Verification items for this drawing (mm, ordinates from the low corner). Give positions to 0.01 mm unless a question says otherwise; leave off trailing zeros. Write each loop counter-clockwise with the first axis right and the second up, starting at its lowest first coordinate (ties: lowest second). Pieces come first, ordered by that corner, then holes. Notation, with made-up numbers: (27.5, 45.25) -> (78.5, 45.25) arc R22 cw to (78.5, 58.25) -> close; hole circle Ø6 at (64.5, -6). An arc over 180 degrees is marked (long way). Answer as a JSON object with one key per item and string values.
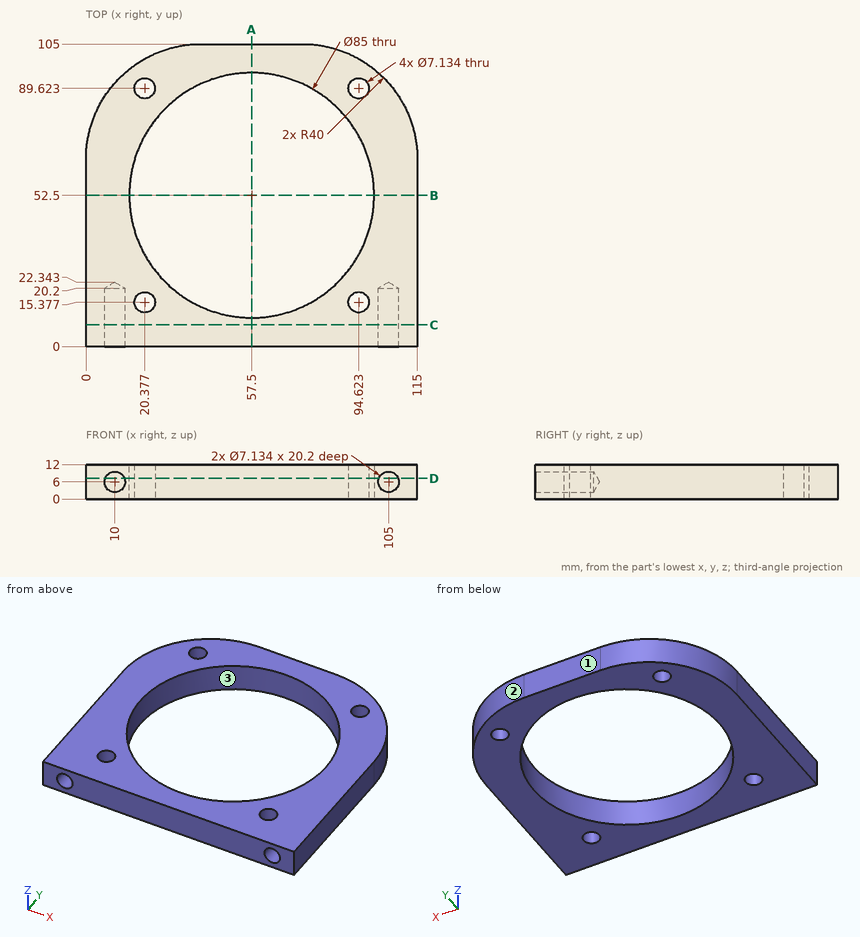
1. Mould release check, pull along X, two halves, no side actions. Record for the marked faces 1, 2 and 3: released by +X, released by -X, zero draft, split by the parting line, or undercut.
Determined:
{"face 1": "zero draft", "face 2": "released by +X", "face 3": "undercut"}
2. Scan lines: L1, parallel to X at y = 7.75, z = 6; L2, parallel to Y at x = 18.5, z = 10.5 (1 decimal); L3, parallel to X at y = 6, z = 7.5. Record each from-to range of solid material in increasing order. Write a range as [from, to].
Determined:
{"L1": "[0, 6.43], [13.57, 101.43], [108.57, 115]", "L2": "[0, 12.3], [18.4, 35.6], [69.4, 86.6], [92.7, 98.7]", "L3": "[0, 6.76], [13.24, 101.76], [108.24, 115]"}
3. Sectioned sample at D-D, the plane z = 7.25. State how many separate pieces and enclosed holes the cut face has, plus the area to 3 significant figures.
Determined:
{"separate pieces": "1", "enclosed holes": "5", "area": "5,270 mm^2"}
4. Sectioned sample at B-B, the plane y = 52.5. Enter the section's corners in (x, z), plus the area to 3 significant figures.
Determined:
{"outline": "(0, 0) -> (15, 0) -> (15, 12) -> (0, 12) -> close; (100, 0) -> (115, 0) -> (115, 12) -> (100, 12) -> close", "area": "360 mm^2"}
5. Sectioned sample at A-A, the plane x = 57.5. Enter the section's corners in (y, z), plus the area to 3 significant figures.
Determined:
{"outline": "(0, 0) -> (10, 0) -> (10, 12) -> (0, 12) -> close; (95, 0) -> (105, 0) -> (105, 12) -> (95, 12) -> close", "area": "240 mm^2"}
6. Sectioned sample at C-C, the plane y = 7.5. Enter the section's corners in (x, z).
Determined:
{"outline": "(0, 0) -> (115, 0) -> (115, 12) -> (0, 12) -> close; hole circle Ø7.13 at (10, 6); hole circle Ø7.13 at (105, 6)"}
7. Go/stop test with flat-tipped pins: P1, Ø2, axis at y = 80, z = 10, coming from the +X side; P2, Ø2, axis at x = 23.5, y = 13.5, coming from the -Z side; P3, Ø6, axis at y = 76.5, z = 7.5, coming from the -X side. Record where each tip stops, or that it passes through.
Determined:
{"P1": "x = 112.47", "P2": "z = 0", "P3": "x = 0.91"}
